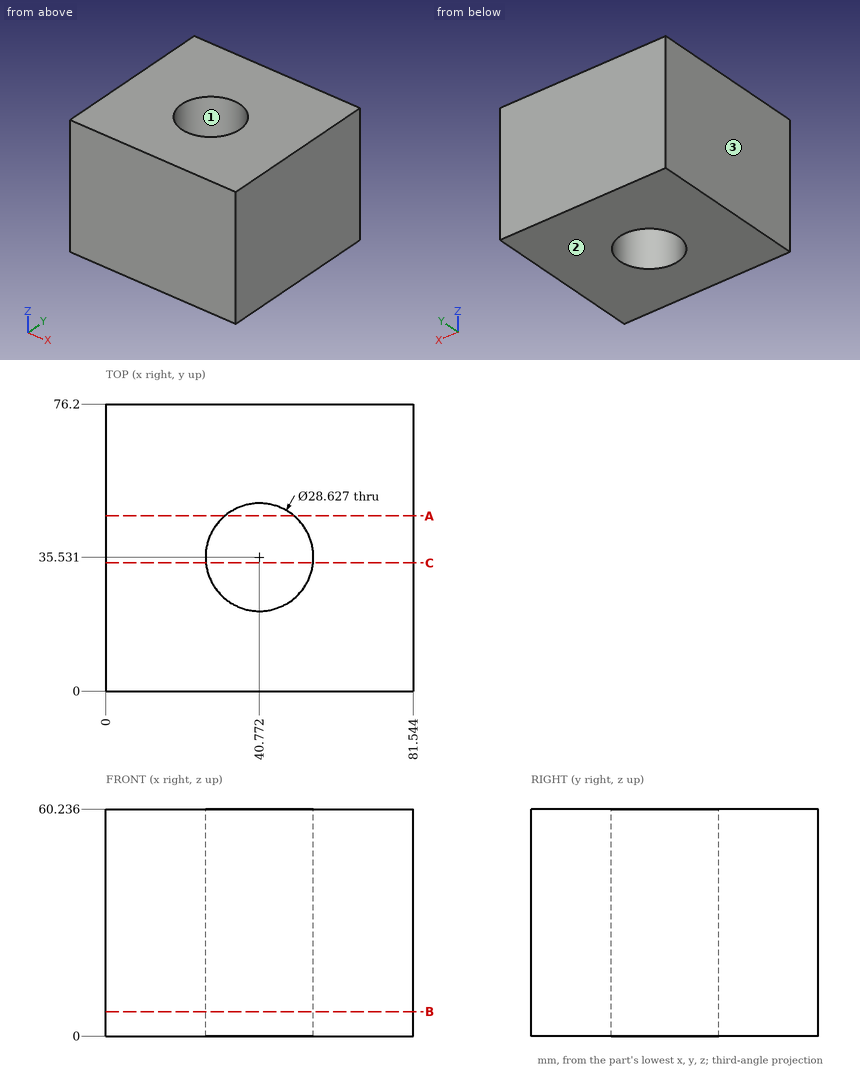
Study the drawing (mm; zero at the part's minimum x, y, z) and answer. Coordinates: 2 decimals unless noted, no trailing zeros. Write each loop counter-clockwise with the first axis right and the second up, starting at its lowest first coordinate (ties: lowest second). Pieces come first, ordered by that corner, then holes. Notation, with made-up numbers: M 33.25,82.5 L 78.25,82.5 A15 ccw 78.25,108.5 Z; hole C 70.5,89 d10. An arc over 180 degrees is marked long. Use a Markdown table: item, result. Add a question column.
1. Given P1, Ø12, axis at x = 22.5, z = 16.5, coming from the -Y side, flat-ended and moving along its own axis, determine where the tip first touches the part or whether it passes through.
2. Straight lines are drawn through the part: line 1 along X through (y, z) = (36, 51.5); line 2 along Y through (x, z) = (31, 6.5) (1 decimal); line 3 along X through (y, z) = (44, 41) (1 decimal). For each, find the intervals that lie inside material, in ascending order. Write a range as [from, to].
3. Section B-B (z = 6.5) is taken. Give the vertices of the cut face in (x, y) (1 decimal), plus the area to 3 significant figures.
4. Section A-A (y = 46.5) is taken. Give the vertices of the cut face in (x, z) (1 decimal).
5. For a pull along X with two mould halves and no side action, classify the marked faces 1, 2 and 3 as +X half, -X half, draft (parallel to the pull), parting line (faces both ways), or undercut.
6. Section C-C (y = 34) is taken. Give the vertices of the cut face in (x, z) (1 decimal).
Data:
| question | item | result |
|---|---|---|
| 1 | P1 | stops at y = 0 |
| 2 | line 1 | x = [0, 26.47], [55.08, 81.54] |
| 2 | line 2 | y = [0, 25.1], [46, 76.2] |
| 2 | line 3 | x = [0, 29.2], [52.3, 81.5] |
| 3 | outline | M 0,0 L 81.5,0 L 81.5,76.2 L 0,76.2 Z; hole C 40.8,35.5 d28.6 |
| 3 | area | 5,570 mm2 |
| 4 | outline | M 0,0 L 31.6,0 L 31.6,60.2 L 0,60.2 Z; M 50,0 L 81.5,0 L 81.5,60.2 L 50,60.2 Z |
| 5 | face 1 | undercut |
| 5 | face 2 | draft |
| 5 | face 3 | -X half |
| 6 | outline | M 0,0 L 26.5,0 L 26.5,60.2 L 0,60.2 Z; M 55,0 L 81.5,0 L 81.5,60.2 L 55,60.2 Z |
